Check sheet for the modelled part. Datum: model origin and axes. Units: mm. A direction names the side the tool comes from. Round coordinates to 2 decimals unless told otherwise and drop trailing zeros. Write each loop counter-clockwise with the first axis right and the second up, starting at its lowest first coordinate (ties: lowest second). Pieces come first, ordered by that corner, then holes. Notation, with made-up numbers: (45, 76.5) - (55, 76.5) arc R6 ccw to (55, 87.5) - close; hole circle Ø8 at (36, 40). An arc over 180 degrees is marked (long way). Use one line per item in the form item = value. Start each with the question number.
1) Section check D-D (y = 14). Record the boundary of the cut face in (x, z), then the cut area to 3 significant figures.
2) Gauge pin test, flat ends, axial feed: P1, Ø1.5, axis at y = 3, z = -14, coming from the +X side; P2, Ø2.5, axis at x = -12.5, y = 7.5, coming from the -Z side; P3, Ø4.5, axis at y = 10, z = -16, coming from the -X side; P4, Ø2, axis at x = -5.5, y = 7, coming from the -Z side. Record the tip position at first contact, or that the pin passes through.
3) Section check B-B (y = 7.5). Record the boundary of the cut face in (x, z).
4) Draft check along Z on faces 1 (the face through (-2.5, 0, -7)), 2 (the face through (-3.6, 7.6, -3.57)), 3 (the face through (-1.48, 5.98, -14.16)), 4 (the face through (-2, 8, -1)). Enter one of: +Z half, -Z half, draft (parallel to the pull), parting line (faces both ways), or undercut.
5) Scan lines: probe 1 along Y at (x, z) = (-12.5, -2.25); probe 2 along X at (y, z) = (2, -8.75). Record each from-to range of solid material in increasing order.
6) Section check A-A (z = -12.5). Record the boundary of the cut face in (x, y).
7) Set-up check for faces 5 (the face through (-14.3, 5.7, -3)), 6 (the face through (-2, 7, -20)): record each of +Z, -Z, +X, -X, +Y, -Y from which the full face is reachable in a straight line by a thin tool's end or side.
8) Section check C-C (x = -12.5). Record the boundary of the cut face in (y, z), then the cut area to 3 significant figures.
Autodesk Inventor part; units mm, degrees
ref_plane "YZ Plane" through (0, 0, 0) normal (1, 0, 0) x (0, 1, 0)
ref_plane "XZ Plane" through (0, 0, 0) normal (0, 1, 0) x (-1, 0, 0)
ref_plane "XY Plane" through (0, 0, 0) normal (0, 0, 1) x (1, 0, 0)
sketch "Sketch1" plane through (0, 0, 0) normal (0, 1, 0) x (-1, 0, 0)
  line L0 (0, 0) -> (20, 0)
  line L1 (20, 0) -> (20, -3)
  line L2 (20, -3) -> (0, -3)
  line L3 (0, -3) -> (0, 0)
  line L4 (0, 0) -> (3, 0)
  line L5 (3, 0) -> (3, -20)
  line L6 (3, -20) -> (0, -20)
  line L7 (0, -20) -> (0, 0)
  dimension "d0" = 3
  dimension "d1" = 3
  dimension "d2" = 20
  dimension "d3" = 20
extrude "Extrusion1" add sketch "Sketch1" along normal blind 15
fillet "Fillet1" radius 2 1 edges at (-3, 7.5, -3)
fillet "Fillet2" radius 5 1 edges at (0, 7.5, 0)
sketch "Sketch2" plane through (-3, 0, -20) normal (-1, 0, 0) x (0, 0, 1)
  line L0 (0, 15) -> (15, 15)
  line L1 (0, 0) -> (15, 0)
  line L2 (0, 0) -> (0, 15)
  point P0 (20, 0)
  point P1 (7.5, 7.5)
  dimension "d9" = 7.5
  dimension "d29" = 7.5
hole "Hole1" at (-3, 7.5, -12.5) direction (1, 0, 0) diameter 4.5 end through all
sketch "Sketch3" plane through (-20, 0, -3) normal (0, 0, -1) x (-1, 0, 0)
  line L0 (-15, 15) -> (0, 15)
  line L1 (-15, 0) -> (0, 0)
  line L2 (0, 0) -> (0, 15)
  point P0 (-20, 0)
  point P1 (-7.5, 7.5)
  dimension "d20" = 7.5
  dimension "d30" = 7.5
hole "Hole2" at (-12.5, 7.5, -3) direction (0, 0, 1) diameter 4.5 end through all
equation "\"d1\" = d0"
equation "\"d3\" = d2"
properties part number "Pancake_Angle Bracket" material "Aluminum 6061"
Results are:
q1.outline = (-20, -3) - (-5, -3) arc R2 cw to (-3, -5) - (-3, -20) - (0, -20) - (0, -5) arc R5 ccw to (-5, 0) - (-20, 0) - close
q1.area = 106 mm²
q2.P1 = 0
q2.P2 = through
q2.P3 = -3
q2.P4 = -3.06
q3.outline = (-20, -3) - (-14.75, -3) - (-14.75, 0) - (-20, 0) - close; (-10.25, -3) - (-5, -3) arc R2 cw to (-3, -5) - (-3, -10.25) - (0, -10.25) - (0, -5) arc R5 ccw to (-5, 0) - (-10.25, 0) - close; (-3, -20) - (0, -20) - (0, -14.75) - (-3, -14.75) - close
q4.face_1 = draft
q4.face_2 = -Z half
q4.face_3 = undercut
q4.face_4 = +Z half
q5.probe_1 = 0 to 5.25, 9.75 to 15
q5.probe_2 = -3 to 0
q6.outline = (-3, 0) - (0, 0) - (0, 5.25) - (-3, 5.25) - close; (-3, 9.75) - (0, 9.75) - (0, 15) - (-3, 15) - close
q7.face_5 = -Z, -X, +Y, -Y
q7.face_6 = -Z, +X, -X, +Y, -Y
q8.outline = (0, -3) - (5.25, -3) - (5.25, 0) - (0, 0) - close; (9.75, -3) - (15, -3) - (15, 0) - (9.75, 0) - close
q8.area = 31.5 mm²
